Build history of the part. All positions in model axes, mm. Round coordinates to 2 decimals unless told otherwise and drop trailing zeros. Loops run counter-clockwise (first coordinate to the right, second up) from the corner with the lowest first, then second, coordinate; pieces in that order, holes last.
from build123d import *

# Parameters (mm, degrees)
SKETCH1_R             = 57.15
SKETCH1_W             = 25.527
SKETCH1_H             = 25.527
BOSS_EXTRUDE1_DEPTH   = 6.35
F_6_CLEARANCE_HOLE1_D = 3.7973
CIRPATTERN1_COUNT     = 12
SKETCH4_R             = 3.4925
CUT_EXTRUDE1_DEPTH    = 3.048
CIRPATTERN2_COUNT     = 12


with BuildPart() as part:
    # Sketch1 → Boss-Extrude1 (new body)
    with BuildSketch(Plane.XY):
        Circle(SKETCH1_R)
        Rectangle(SKETCH1_W, SKETCH1_H, mode=Mode.SUBTRACT)
    extrude(amount=BOSS_EXTRUDE1_DEPTH)

    # #6 Clearance Hole1 (through all)
    with Locations(Plane(origin=(0, 0, 0), x_dir=(-1, 0, 0), z_dir=(0, 0, -1))):
        with Locations((35.921024484, 35.921024484)):
            f_6_clearance_hole1 = Hole(F_6_CLEARANCE_HOLE1_D / 2)

    # CirPattern1: #6 Clearance Hole1 ×12 about axis
    cirpattern1_axis = Axis((0, 0, 0), (0, 0, 1))
    for i in range(1, CIRPATTERN1_COUNT):
        add(f_6_clearance_hole1.rotate(cirpattern1_axis, i * 360 / CIRPATTERN1_COUNT), mode=Mode.SUBTRACT)

    # Sketch4 → Cut-Extrude1 (cut)
    with BuildSketch(Plane(origin=(0, 0, 0), x_dir=(-1, 0, 0), z_dir=(0, 0, -1))):
        with Locations((35.921024484, 35.921024484)):
            Circle(SKETCH4_R)
    cut_extrude1 = extrude(amount=-CUT_EXTRUDE1_DEPTH, mode=Mode.SUBTRACT)

    # CirPattern2: Cut-Extrude1 ×12 about axis
    cirpattern2_axis = Axis((0, 0, 0), (0, 0, 1))
    for i in range(1, CIRPATTERN2_COUNT):
        add(cut_extrude1.rotate(cirpattern2_axis, i * 360 / CIRPATTERN2_COUNT), mode=Mode.SUBTRACT)


solid = part.part
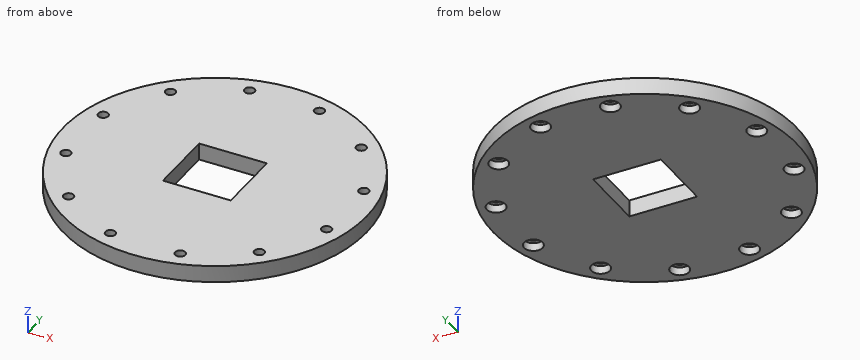
(1) Slice it at C-C on z = 2. Count the separate pieces of the cut face and the enclosed holes in it, plus the area to 3 significant figures.
Responses:
separate pieces: 1
enclosed holes: 13
area: 9,150 mm2
(2) Slice it at D-D on x = 42. List the corners of the cut face in (y, z), plus the area to 3 significant figures.
Responses:
outline: (-38.76, 0) - (38.76, 0) - (38.76, 6.35) - (-38.76, 6.35) - close
area: 492 mm2
(3) Probe line 1 (X direction, y = 1.5, z = 1); line 2 (X direction, y = -48, z = 5); line 3 (X direction, y = 35.5, z = 3.5). List the from-to ranges inside material, lowest first.
Responses:
line 1: x = -57.13 to -12.76, 12.76 to 57.13
line 2: x = -31.02 to -14.72, -11.58 to 11.58, 14.72 to 31.02
line 3: x = -44.79 to -37.77, -34.07 to 34.07, 37.77 to 44.79
(4) Slice it at A-A on x = 0. List the corners of the cut face in (y, z), plus the area to 3 significant figures.
Responses:
outline: (-57.15, 0) - (-12.76, 0) - (-12.76, 6.35) - (-57.15, 6.35) - close; (12.76, 0) - (57.15, 0) - (57.15, 6.35) - (12.76, 6.35) - close
area: 564 mm2
(5) Pin check, flat tips, straight feed: P1, Ø6, axis at x = 49.07, y = -13.15, coming from the -Z side; P2, Ø2, axis at x = 44.5, z = 4, coming from the -Y side. Stop position of each tip, or through.
Responses:
P1: stops at z = 3.05
P2: stops at y = -37.07
